Read the model definition and answer for the solid it produces. Units are mm, in the model's axes. Give positions to 0.01 mm unless a question says otherwise; leave off trailing zeros. Order: outer loops, then holes, each group sorted by start corner. A loop starts at its lowest first (then second) coordinate and runs counter-clockwise, first axis right, second up. Notation, with made-up numbers: (63, 26) - (82, 26) arc R18 cw to (82, 55) - close; hole circle Ø11 at (-8.5, 64). An arc over 180 degrees is marked (long way). One line per item, written item: value. Start each with the question number.
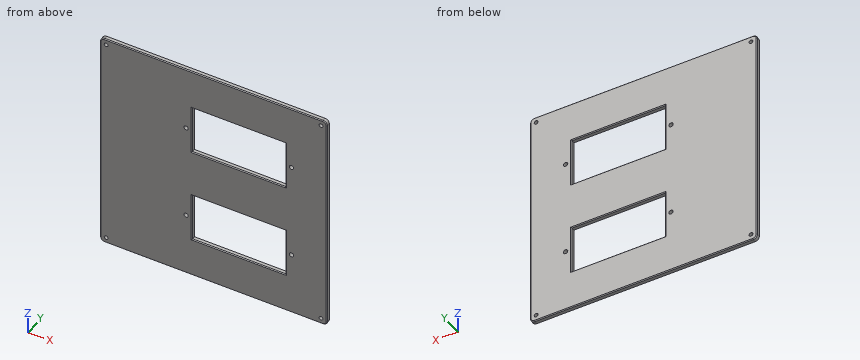
```python
from build123d import *

# Parameters (mm, degrees)
SKETCH1_W           = 268.29
SKETCH1_H           = 268.29
SKETCH1_R           = 2.25
SKETCH1_R_2         = 2.55
SKETCH1_W_2         = 110.6
SKETCH1_H_2         = 57.65
BOSS_EXTRUDE1_DEPTH = 5.8
FILLET1_R           = 5
CHAMFER1_SIZE       = 1


with BuildPart() as part:
    # Sketch1 → Boss-Extrude1 (new body)
    with BuildSketch(Plane(origin=(0, 0, 0), x_dir=(1, 0, 0), z_dir=(0, 1, 0))):
        Rectangle(SKETCH1_W, SKETCH1_H)
        with Locations(Location((-127.095, 127.095, 0), (0, 0, 270))):
            Circle(SKETCH1_R, mode=Mode.SUBTRACT)
        with Locations(Location((127.095, 127.095, 0), (0, 0, 270))):
            Circle(SKETCH1_R, mode=Mode.SUBTRACT)
        with Locations(Location((127.095, -127.095, 0), (0, 0, 270))):
            Circle(SKETCH1_R, mode=Mode.SUBTRACT)
        with Locations(Location((-127.095, -127.095, 0), (0, 0, 270))):
            Circle(SKETCH1_R, mode=Mode.SUBTRACT)
        with Locations(Location((-32.505, 58.02, 0), (0, 0, 270))):
            Circle(SKETCH1_R_2, mode=Mode.SUBTRACT)
        with Locations(Location((-32.505, -57.17, 0), (0, 0, 270))):
            Circle(SKETCH1_R_2, mode=Mode.SUBTRACT)
        with Locations(Location((92.195, -57.17, 0), (0, 0, 270))):
            Circle(SKETCH1_R_2, mode=Mode.SUBTRACT)
        with Locations(Location((92.195, 58.02, 0), (0, 0, 270))):
            Circle(SKETCH1_R_2, mode=Mode.SUBTRACT)
        with Locations((29.845, 58.02)):
            Rectangle(SKETCH1_W_2, SKETCH1_H_2, mode=Mode.SUBTRACT)
        with Locations((29.845, -57.17)):
            Rectangle(SKETCH1_W_2, SKETCH1_H_2, mode=Mode.SUBTRACT)
    extrude(amount=BOSS_EXTRUDE1_DEPTH)

    # Fillet1
    fillet1_edges = [part.edges().sort_by_distance(p)[0] for p in [
        (134.145, 2.9, 134.145),
        (-134.145, 2.9, 134.145),
        (-134.145, 2.9, -134.145),
        (134.145, 2.9, -134.145),
    ]]
    fillet(fillet1_edges, radius=FILLET1_R)

    # Chamfer1
    chamfer1_edges = [part.edges().sort_by_distance(p)[0] for p in [
        (85.145, 0, 57.17),
        (29.845, 0, 28.345),
        (-25.455, 0, 57.17),
        (29.845, 0, 85.995),
        (85.145, 5.8, 57.17),
        (29.845, 5.8, 28.345),
        (-25.455, 5.8, 57.17),
        (29.845, 5.8, 85.995),
        (85.145, 0, -58.02),
        (29.845, 0, -86.845),
        (-25.455, 0, -58.02),
        (29.845, 0, -29.195),
        (85.145, 5.8, -58.02),
        (29.845, 5.8, -86.845),
        (-25.455, 5.8, -58.02),
        (29.845, 5.8, -29.195),
        (134.145, 0, 0),
        (134.145, 5.8, 0),
        (0, 0, 134.145),
        (-134.145, 0, 0),
        (0, 0, -134.145),
        (-132.680533906, 0, 132.680533906),
        (-132.680533906, 0, -132.680533906),
        (132.680533906, 0, -132.680533906),
        (132.680533906, 0, 132.680533906),
        (0, 5.8, 134.145),
        (0, 5.8, -134.145),
        (-134.145, 5.8, 0),
        (-132.680533906, 5.8, 132.680533906),
        (-132.680533906, 5.8, -132.680533906),
        (132.680533906, 5.8, -132.680533906),
        (132.680533906, 5.8, 132.680533906),
    ]]
    chamfer(chamfer1_edges, length=CHAMFER1_SIZE)


solid = part.part
```
1) This flat-tipped pin is pushed along its axis until it touches: pin 1 (3.5 mm diameter, centred on x = 127.095, z = 127.095, fed in from -Y). Where does it stop, or does it pass through?
2) Section B-B on z = 75 is taken. Write down the section's boundary in (x, y) (3 decimals).
3) Find the intervals of material crossed by probe 1 along X at (y, z) = (3.3, 57.17) (3 decimals); probe 2 along Z at (x, y) = (18, 4.4) (3 decimals); probe 3 along Z at (x, y) = (90, 3.7) (3 decimals), in increasing order. Write a range as from..to.
4) Section A-A on x = 47 is taken. Write down the section's boundary in (y, z) (3 decimals).
5) Section C-C on y = 2.75 is taken. Give the number of separate pieces and of enclosed holes in the cut face, plus the area to 3 significant figures.
Solved:
1. pin 1: passes through
2. outline: (-134.145, 1) - (-133.145, 0) - (-26.455, 0) - (-25.455, 1) - (-25.455, 4.8) - (-26.455, 5.8) - (-133.145, 5.8) - (-134.145, 4.8) - close; (85.145, 1) - (86.145, 0) - (133.145, 0) - (134.145, 1) - (134.145, 4.8) - (133.145, 5.8) - (86.145, 5.8) - (85.145, 4.8) - close
3. probe 1: x = -134.145..-35.055, -29.955..-25.455, 85.145..89.645, 94.745..134.145
3. probe 2: z = -134.145..-86.845, -29.195..28.345, 85.995..134.145
3. probe 3: z = -134.145..-59.318, -56.722..55.872, 58.468..134.145
4. outline: (0, -133.145) - (1, -134.145) - (4.8, -134.145) - (5.8, -133.145) - (5.8, -87.845) - (4.8, -86.845) - (1, -86.845) - (0, -87.845) - close; (0, -28.195) - (1, -29.195) - (4.8, -29.195) - (5.8, -28.195) - (5.8, 27.345) - (4.8, 28.345) - (1, 28.345) - (0, 27.345) - close; (0, 86.995) - (1, 85.995) - (4.8, 85.995) - (5.8, 86.995) - (5.8, 133.145) - (4.8, 134.145) - (1, 134.145) - (0, 133.145) - close
5. separate pieces: 1
5. enclosed holes: 10
5. area: 59,100 mm2
